Can you work these out from the drawing? Everything is in mm from the part's minimum corner. Round coordinates to 2 decimals unless told otherwise and drop trailing zeros. Write each loop counter-clockwise with the first axis right and the second up, starting at its lowest first coordinate (ties: lowest second). Pieces come first, ordered by that corner, then holes.
Q1. Please list where these lines run through material, in increasing order: line 1 along Z through (x, y) = (160, 4.1); line 2 along Z through (x, y) = (133, 1.1) (1 decimal).
Q2. If we section it at B-B (x = 214.5): Please give me the cut outline in (y, z), plus the area to 3 significant figures.
Q3. I'm going to push a flat-ended pin straight in: pin 1 Ø1 at (x, y) = (314, 5) entering from -Z. Where does the tip first touch, or does it pass through?
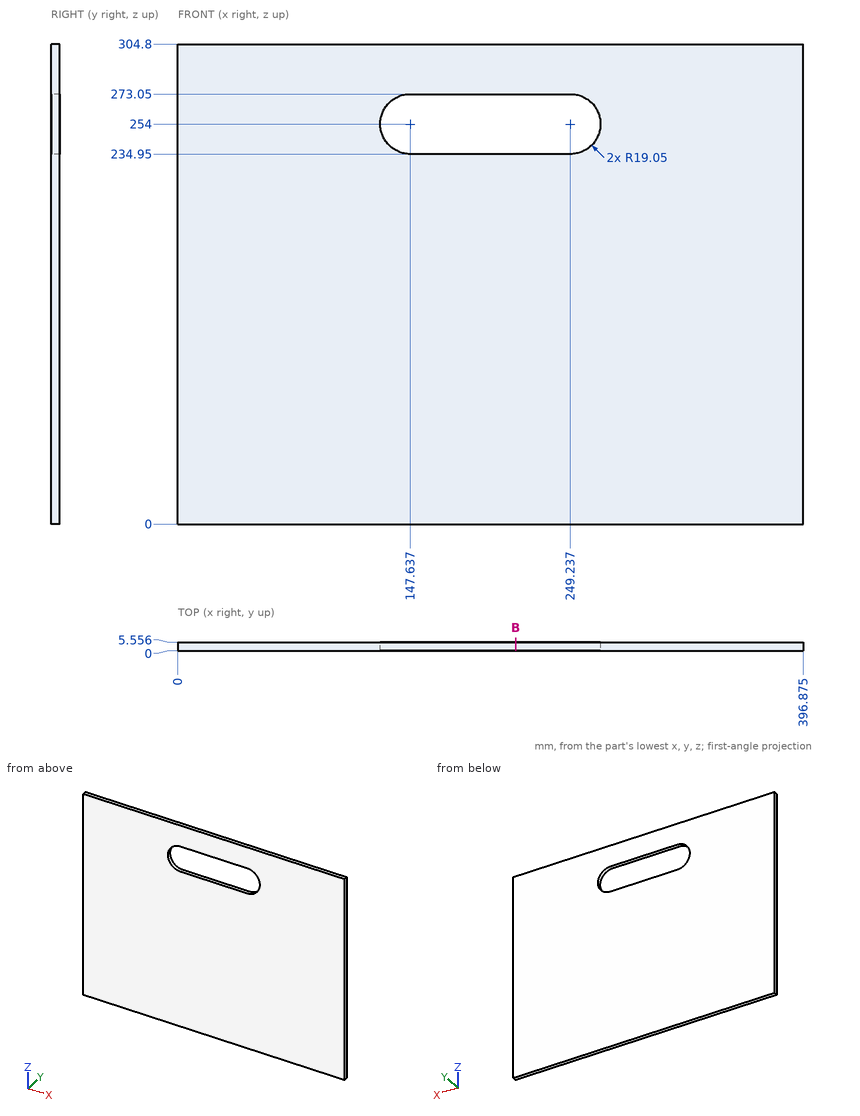
A:
1. line 1: z = 0 to 234.95, 273.05 to 304.8
1. line 2: z = 0 to 241.8, 266.2 to 304.8
2. outline: (0, 0) - (5.56, 0) - (5.56, 234.95) - (0, 234.95) - close; (0, 273.05) - (5.56, 273.05) - (5.56, 304.8) - (0, 304.8) - close
2. area: 1,480 mm2
3. pin 1: stops at z = 0
